Can you work these out from the model? Positions are in its coordinate system, mm. A direction names the side the tool comes from. Round coordinates to 2 decimals unless told otherwise and drop trailing zeros. Order: outer loops, then holes, each group sorted by start corner. A loop starts at its lowest first (then second) coordinate and runs counter-clockwise, first axis right, second up. Notation, with made-up numbers: (-28.75, 32.25) - (30.25, 32.25) arc R30 cw to (30.25, 56.25) - close; hole circle Ø2 at (41, 85). An arc over 180 degrees is marked (long way). Write item = value, one per line.
from build123d import *

# Parameters (mm, degrees)
IZIM1_W               = 64
IZIM1_H               = 54
IZIM1_W_2             = 60
IZIM1_H_2             = 50
EKSTR_ZYON_NCE1_DEPTH = 50
KES_EKSTR_ZYON1_REACH = 98.437
IZIM2_R               = 4
IZIM2_R_2             = 2


with BuildPart() as part:
    # Çizim1 → Ekstrüzyon-İnce1 (new body)
    with BuildSketch(Plane.XY):
        with Locations((30, 25)):
            Rectangle(IZIM1_W, IZIM1_H)
        with Locations((30, 25)):
            Rectangle(IZIM1_W_2, IZIM1_H_2, mode=Mode.SUBTRACT)
    extrude(amount=EKSTR_ZYON_NCE1_DEPTH)

    # Çizim2 → Kes-Ekstrüzyon1 (cut, up to next)
    with BuildSketch(Plane.ZY.offset(2), mode=Mode.PRIVATE) as kes_ekstr_zyon1_sk1:
        with Locations((25, 25)):
            Circle(IZIM2_R)
    kes_ekstr_zyon1_tool1 = extrude(kes_ekstr_zyon1_sk1.sketch, amount=-KES_EKSTR_ZYON1_REACH, mode=Mode.PRIVATE) & part.part
    # Çizim2 → Kes-Ekstrüzyon1 (cut, up to next)
    with BuildSketch(Plane.ZY.offset(2), mode=Mode.PRIVATE) as kes_ekstr_zyon1_sk2:
        with Locations((33, 25)):
            Circle(IZIM2_R_2)
    kes_ekstr_zyon1_tool2 = extrude(kes_ekstr_zyon1_sk2.sketch, amount=-KES_EKSTR_ZYON1_REACH, mode=Mode.PRIVATE) & part.part
    # Çizim2 → Kes-Ekstrüzyon1 (cut, up to next)
    with BuildSketch(Plane.ZY.offset(2), mode=Mode.PRIVATE) as kes_ekstr_zyon1_sk3:
        with Locations(Location((17, 25, 0), (0, 0, 180))):
            Circle(IZIM2_R_2)
    kes_ekstr_zyon1_tool3 = extrude(kes_ekstr_zyon1_sk3.sketch, amount=-KES_EKSTR_ZYON1_REACH, mode=Mode.PRIVATE) & part.part
    # Çizim2 → Kes-Ekstrüzyon1 (cut, up to next)
    with BuildSketch(Plane.ZY.offset(2), mode=Mode.PRIVATE) as kes_ekstr_zyon1_sk4:
        with Locations((25, 33)):
            Circle(IZIM2_R_2)
    kes_ekstr_zyon1_tool4 = extrude(kes_ekstr_zyon1_sk4.sketch, amount=-KES_EKSTR_ZYON1_REACH, mode=Mode.PRIVATE) & part.part
    # Çizim2 → Kes-Ekstrüzyon1 (cut, up to next)
    with BuildSketch(Plane.ZY.offset(2), mode=Mode.PRIVATE) as kes_ekstr_zyon1_sk5:
        with Locations(Location((25, 17, 0), (0, 0, 180))):
            Circle(IZIM2_R_2)
    kes_ekstr_zyon1_tool5 = extrude(kes_ekstr_zyon1_sk5.sketch, amount=-KES_EKSTR_ZYON1_REACH, mode=Mode.PRIVATE) & part.part
    add(kes_ekstr_zyon1_tool1.solids().sort_by_distance((-2, 25, 25))[0], mode=Mode.SUBTRACT)
    add(kes_ekstr_zyon1_tool2.solids().sort_by_distance((-2, 25, 33))[0], mode=Mode.SUBTRACT)
    add(kes_ekstr_zyon1_tool3.solids().sort_by_distance((-2, 25, 17))[0], mode=Mode.SUBTRACT)
    add(kes_ekstr_zyon1_tool4.solids().sort_by_distance((-2, 33, 25))[0], mode=Mode.SUBTRACT)
    add(kes_ekstr_zyon1_tool5.solids().sort_by_distance((-2, 17, 25))[0], mode=Mode.SUBTRACT)


solid = part.part
(1) If I drill on line 1 (Y direction, x = -1, z = 25); line 2 (Y direction, x = 18, z = 45); line 3 (X direction, y = 14.5, z = 36), over which ranges is the centre line in solid material (lowest first)? Write a range as from..to.
Computed:
line_1 = -2..15, 19..21, 29..31, 35..52
line_2 = -2..0, 50..52
line_3 = -2..0, 60..62
(2) Thinking about a two-plate mould opening in Z: for faces 4 (the face through (-2, 25, 30)), 5 (the face through (-1, 26.2, 18.6)), 6 (the face through (27, -1, 0)), which applies, +Z half, -Z half, draft (parallel to the pull), parting line (faces both ways), or undercut?
Computed:
face_4 = draft
face_5 = undercut
face_6 = -Z half
(3) If we section it at C-C (x = 14): Write out the boundary of the cut face in (y, z).
Computed:
outline = (-2, 0) - (0, 0) - (0, 50) - (-2, 50) - close; (50, 0) - (52, 0) - (52, 50) - (50, 50) - close
(4) On a 3-axis mill with a long thin cutter (end or side, diameter ignored), from which of +Z, -Z, +X, -X, +Y, -Y can I reach the whole of each face in a straight line? I mean faces 1 (the face through (-1, 15, 25)), 2 (the face through (62, 25, 25)), 3 (the face through (30, 0, 25)). Say none if no direction works.
Computed:
face_1 = -X
face_2 = +Z, -Z, +X, +Y, -Y
face_3 = +Z, -Z
(5) Will this pin go through, and if not, where does the flat tip stop? P1, Ø10, axis at x = 8, y = 5.5, coming from the -Z side.
Computed:
P1 = through
(6) If we section it at B-B (y = 8): Write out the boundary of the cut face in (x, z).
Computed:
outline = (-2, 0) - (0, 0) - (0, 50) - (-2, 50) - close; (60, 0) - (62, 0) - (62, 50) - (60, 50) - close
(7) If we section it at D-D (z = 37): Write out the boundary of the cut face in (x, y).
Computed:
outline = (-2, -2) - (62, -2) - (62, 52) - (-2, 52) - close; hole (0, 0) - (60, 0) - (60, 50) - (0, 50) - close
(8) If we section it at A-A (z = 25): Write out the boundary of the cut face in (x, y), plus the area to 3 significant figures.
Computed:
outline = (-2, -2) - (62, -2) - (62, 52) - (-2, 52) - (-2, 35) - (0, 35) - (0, 50) - (60, 50) - (60, 0) - (0, 0) - (0, 15) - (-2, 15) - close; (-2, 19) - (0, 19) - (0, 21) - (-2, 21) - close; (-2, 29) - (0, 29) - (0, 31) - (-2, 31) - close
area = 424 mm^2
